For this review, take the finished solid that the model builds, in its own axes (mm). Round coordinates to 2 decimals unless told otherwise and drop trailing zeros. One line per question, with ' | ' between items. Start each with the question number.
1. Consider section A-A (y = -18.6). Count the separate pieces of the cut face and the enclosed holes in it, and give its area (3 significant figures).
2. For pin 1 Ø2 at (y, z) = (-18.5, -21.5) entering from -X; pin 2 Ø5 at (x, z) = (-24.01, 7.36) entering from -Y; pin 3 Ø1.5 at (x, y) = (-21.5, -18.5) entering from -Z; pin 4 Ø1 at (y, z) = (-17, -22.5) entering from -X, all flat-tipped, find the tip position at first contact; note any pin that passes through.
3. Wall thickness on line 1 along Z through (x, y) = (46, -16.5); line 2 along X through (y, z) = (-17.35, 0); line 3 along Z through (x, y) = (44.5, -17.3): over which ranges is each line inside the solid? List them lowest first.
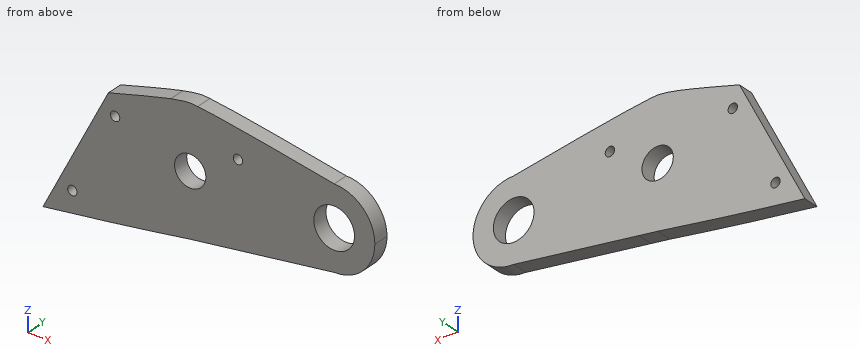
```python
from build123d import *

# Parameters (mm, degrees)
BOSS_EXTRUDE1_DEPTH      = 20
BOSS_EXTRUDE1_DEPTH_BACK = 20
SKETCH1_R                = 5
SKETCH1_R_2              = 6.5
CUT_EXTRUDE4_DEPTH       = 35
SKETCH6_R                = 1.5
CUT_EXTRUDE5_DEPTH       = 10
CUT_EXTRUDE6_DEPTH       = 50


with BuildPart() as part:
    # Sketch1 → Boss-Extrude1 (new, two sides: drawn at the far end of the back side and taken through both)
    # profile 1 of 5: a face of its own
    with BuildSketch(Plane(origin=(0, 0, 0), x_dir=(1, 0, 0), z_dir=(0, 1, 0)).offset(-BOSS_EXTRUDE1_DEPTH_BACK)):
        with BuildLine():
            add(Edge.make_bspline(
                [(-328.284271247, 28.284271247), (-322.910070204, 33.658472291), (-311.873452078, 37.427029787), (-296.732235412, 39.86629798)],
                knots=[0, 0, 0, 0, 0.1900067, 0.1900067, 0.1900067, 0.1900067], degree=3))
            ThreePointArc((-328.284271247, 28.284271247), (-328.284271247, -28.284271247), (-271.715728753, -28.284271247))
            ThreePointArc((-271.715728753, -28.284271247), (-263.0448187, -15.307337295), (-260, 0))
            ThreePointArc((-260, 0), (-270.583078139, 27.104330064), (-296.732235412, 39.86629798))
        make_face()
    # profile 2 of 5: a face of its own
    with BuildSketch(Plane(origin=(0, 0, 0), x_dir=(1, 0, 0), z_dir=(0, 1, 0)).offset(-BOSS_EXTRUDE1_DEPTH_BACK)):
        with BuildLine():
            ThreePointArc((-260, 0), (-263.0448187, -15.307337295), (-271.715728753, -28.284271247))
            add(Edge.make_bspline(
                [(-271.715728753, -28.284271247), (-194.91847241, 48.512985095), (-42.964488834, -10.495172733), (-6.202879594, -19.013791961)],
                knots=[0, 0, 0, 0, 0.930923327, 0.930923327, 0.930923327, 0.930923327], degree=3))
            ThreePointArc((-6.202879594, -19.013791961), (-19.751909265, 3.140394942), (0, 20))
            add(Edge.make_bspline(
                [(-296.732235412, 39.86629798), (-232.185648118, 50.264830728), (-93.046467117, 36.506278231), (0, 20)],
                knots=[0.1900067, 0.1900067, 0.1900067, 0.1900067, 1, 1, 1, 1], degree=3))
            ThreePointArc((-296.732235412, 39.86629798), (-270.583078139, 27.104330064), (-260, 0))
        make_face()
    # profile 3 of 5: a face of its own
    with BuildSketch(Plane(origin=(0, 0, 0), x_dir=(1, 0, 0), z_dir=(0, 1, 0)).offset(-BOSS_EXTRUDE1_DEPTH_BACK)):
        with BuildLine():
            ThreePointArc((0, 20), (-19.751909265, 3.140394942), (-6.202879594, -19.013791961))
            add(Edge.make_bspline(
                [(-6.202879594, -19.013791961), (-3.475082803, -19.645893294), (-1.381533462, -20), (0, -20)],
                knots=[0.930923327, 0.930923327, 0.930923327, 0.930923327, 1, 1, 1, 1], degree=3))
            add(Edge.make_bspline(
                [(0, -20), (0.844585297, -20), (2.387633143, -19.856968751)],
                knots=[0, 0, 0, 0.142944169, 0.142944169, 0.142944169], degree=2))
            ThreePointArc((2.387633143, -19.856968751), (14.9624975, -13.271159278), (20, 0))
            ThreePointArc((20, 0), (16.104446086, 11.859461044), (5.935318374, 19.0990051))
            add(Edge.make_bspline(
                [(0, 20), (0.011302239, 20), (5.935318374, 19.0990051)],
                knots=[0, 0, 0, 0.358766717, 0.358766717, 0.358766717], degree=2))
        make_face()
        with Locations(Location((0, 0, 0), (0, 0, 270))):
            Circle(SKETCH1_R, mode=Mode.SUBTRACT)
    # profile 4 of 5: a face of its own
    with BuildSketch(Plane(origin=(0, 0, 0), x_dir=(1, 0, 0), z_dir=(0, 1, 0)).offset(-BOSS_EXTRUDE1_DEPTH_BACK)):
        with BuildLine():
            add(Edge.make_bspline(
                [(5.935318374, 19.0990051), (16.523469771, 17.488632981), (46, 13)],
                knots=[0.358766717, 0.358766717, 0.358766717, 1, 1, 1], degree=2))
            ThreePointArc((5.935318374, 19.0990051), (16.104446086, 11.859461044), (20, 0))
            ThreePointArc((20, 0), (14.9624975, -13.271159278), (2.387633143, -19.856968751))
            add(Edge.make_bspline(
                [(2.387633143, -19.856968751), (11.639344201, -18.999390814), (46, -13)],
                knots=[0.142944169, 0.142944169, 0.142944169, 1, 1, 1], degree=2))
            ThreePointArc((46, -13), (33, 0), (46, 13))
        make_face()
    # profile 5 of 5: a face of its own
    with BuildSketch(Plane(origin=(0, 0, 0), x_dir=(1, 0, 0), z_dir=(0, 1, 0)).offset(-BOSS_EXTRUDE1_DEPTH_BACK)):
        with BuildLine():
            ThreePointArc((59, 0), (55.192388155, 9.192388155), (46, 13))
            ThreePointArc((46, 13), (33, 0), (46, -13))
            ThreePointArc((46, -13), (55.192388155, -9.192388155), (59, 0))
        make_face()
        with Locations(Location((46, 0, 0), (0, 0, 270))):
            Circle(SKETCH1_R_2, mode=Mode.SUBTRACT)
    extrude(amount=BOSS_EXTRUDE1_DEPTH + BOSS_EXTRUDE1_DEPTH_BACK)

    # Sketch5 → Cut-Extrude4 (cut)
    with BuildSketch(Plane(origin=(0, 20, 0), x_dir=(1, 0, 0), z_dir=(0, 1, 0))):
        Polygon((-47.037049996, 27.527548523), (92.120786702, 16.164640032), (85.724700256, -16.918764701), (-17.262768022, -30.907770073), align=None)
    extrude(amount=-CUT_EXTRUDE4_DEPTH, mode=Mode.SUBTRACT)

    # Sketch6 → Cut-Extrude5 (cut)
    with BuildSketch(Plane(origin=(0, -20, 0), x_dir=(-1, 0, 0), z_dir=(0, -1, 0))):
        with Locations(Location((24.005160607, -7.356928903, 0), (0, 0, 90))):
            Circle(SKETCH6_R)
        with Locations(Location((-15.251108102, -8.960330165, 0), (0, 0, 90))):
            Circle(SKETCH6_R)
        with Locations(Location((37.643080162, 19.408995291, 0), (0, 0, 90))):
            Circle(SKETCH6_R)
    extrude(amount=-CUT_EXTRUDE5_DEPTH, mode=Mode.SUBTRACT)

    # Sketch7 → Cut-Extrude6 (cut)
    with BuildSketch(Plane(origin=(0, 20, 0), x_dir=(1, 0, 0), z_dir=(0, 1, 0))):
        Polygon((-47.037049996, 27.527548523), (-26.137658318, -13.489817144), (-379.595719096, -92.580220424), (-321.505561991, 137.254748988), align=None)
    extrude(amount=-CUT_EXTRUDE6_DEPTH, mode=Mode.SUBTRACT)


solid = part.part
```
Answer block:
1) separate pieces: 1 | enclosed holes: 5 | area: 2,990 mm2
2) pin 1: stops at x = -44.48 | pin 2: stops at y = -20 | pin 3: stops at z = -23.75 | pin 4: stops at x = -44.73
3) line 1: z = -13 to -6.5, 6.5 to 13 | line 2: x = -33.01 to -5, 5 to 39.5, 52.5 to 59 | line 3: z = -13.23 to -6.32, 6.32 to 13.26
